Verification items for the finished model (mm, model axes). Face numbers are marked on the shaded views. A direction names the side the tool comes from. Round coordinates to 2 decimals unless told otherwise and drop trailing zeros. Order: outer loops, then holes, each group sorted by start corner. A loop starts at its lowest first (then second) coordinate and runs counter-clockwise, first axis right, second up. Notation, with made-up numbers: (64.5, -21.5) -> (119.5, -21.5) arc R24 ccw to (119.5, 13.5) -> close; hole circle Ø7 at (81.25, 66). An arc over 180 degrees is marked (long way). Put each result on its own line as item: value.
from build123d import *

# Parameters (mm, degrees)
CROQUIS1_W               = 22
CROQUIS1_H               = 55.2
SALIENTE_EXTRUIR1_DEPTH  = 4
CROQUIS2_W               = 12.1
CROQUIS2_H               = 4
CORTAR_EXTRUIR1_DEPTH    = 9.6
CROQUIS3_W               = 12.1
CROQUIS3_H               = 4
CORTAR_EXTRUIR2_DEPTH    = 9.6
CORTAR_EXTRUIR3_DEPTH    = 16
CORTAR_EXTRUIR4_START    = -16
CORTAR_EXTRUIR4_DEPTH    = 16
CROQUIS9_W               = 11.778481694
CROQUIS9_H               = 4
CORTAR_EXTRUIR5_DEPTH    = 2
CROQUIS11_W              = 4.95
CROQUIS11_H              = 4
SALIENTE_EXTRUIR3_DEPTH  = 2
CROQUIS12_W              = 4
CROQUIS12_H              = 1.8
SALIENTE_EXTRUIR4_DEPTH  = 12.1
CROQUIS13_W              = 4.95
CROQUIS13_H              = 4
SALIENTE_EXTRUIR5_DEPTH  = 2
CROQUIS14_W              = 4
CROQUIS14_H              = 1.8
SALIENTE_EXTRUIR6_DEPTH  = 12.1
CROQUIS17_W              = 4
CROQUIS17_H              = 59.2
SALIENTE_EXTRUIR8_DEPTH  = 15
CROQUIS18_W              = 4
CROQUIS18_H              = 59.2
SALIENTE_EXTRUIR9_DEPTH  = 15
CROQUIS19_R              = 1.75
CORTAR_EXTRUIR6_DEPTH    = 11.5
CROQUIS20_R              = 8.8
CROQUIS20_R_2            = 8.901027098
CORTAR_EXTRUIR7_DEPTH    = 4
CROQUIS22_R              = 10
SALIENTE_EXTRUIR10_DEPTH = 6
CORTAR_EXTRUIR8_DEPTH    = 10
CROQUIS26_R              = 8.901027098
CROQUIS26_R_2            = 8.8
CORTAR_EXTRUIR9_DEPTH    = 2


with BuildPart() as part:
    # Croquis1 → Saliente-Extruir1 (new body)
    with BuildSketch(Plane.XY):
        with Locations((11, 27.6)):
            Rectangle(CROQUIS1_W, CROQUIS1_H)
    extrude(amount=SALIENTE_EXTRUIR1_DEPTH)

    # Croquis2 → Cortar-Extruir1 (cut)
    with BuildSketch(Plane(origin=(0, 55.2, 0), x_dir=(1, 0, 0), z_dir=(0, 1, 0))):
        with Locations((11, -2)):
            Rectangle(CROQUIS2_W, CROQUIS2_H)
    extrude(amount=-CORTAR_EXTRUIR1_DEPTH, mode=Mode.SUBTRACT)

    # Croquis3 → Cortar-Extruir2 (cut)
    with BuildSketch(Plane.XZ):
        with Locations((11, 2)):
            Rectangle(CROQUIS3_W, CROQUIS3_H)
    extrude(amount=-CORTAR_EXTRUIR2_DEPTH, mode=Mode.SUBTRACT)

    # Croquis5 → Cortar-Extruir3 (cut)
    with BuildSketch(Plane.XZ.offset(-9.6)):
        with BuildLine():
            Line((7.4, 4), (14.6, 4))
            ThreePointArc((14.6, 4), (16.401151853, 1.506649462), (17.05, -1.5))
            Line((17.05, -1.5), (4.95, -1.5))
            ThreePointArc((4.95, -1.5), (5.598848147, 1.506649462), (7.4, 4))
        make_face()
    extrude(amount=-CORTAR_EXTRUIR3_DEPTH, mode=Mode.SUBTRACT)

    # Croquis7 → Cortar-Extruir4 (cut)
    with BuildSketch(Plane(origin=(0, 45.6, 0), x_dir=(1, 0, 0), z_dir=(0, 1, 0)).offset(CORTAR_EXTRUIR4_START)):
        with BuildLine():
            Line((4.95, 1.5), (17.05, 1.5))
            ThreePointArc((17.05, 1.5), (16.401151853, -1.506649462), (14.6, -4))
            Line((14.6, -4), (7.4, -4))
            ThreePointArc((7.4, -4), (5.598848147, -1.506649462), (4.95, 1.5))
        make_face()
    extrude(amount=CORTAR_EXTRUIR4_DEPTH, mode=Mode.SUBTRACT)

    # Croquis9 → Cortar-Extruir5 (cut)
    with BuildSketch(Plane(origin=(0, 0, 0), x_dir=(-1, 0, 0), z_dir=(0, 0, -1))):
        with Locations((-11, 27.6)):
            Rectangle(CROQUIS9_W, CROQUIS9_H)
    extrude(amount=-CORTAR_EXTRUIR5_DEPTH, mode=Mode.SUBTRACT)

    # Croquis11 → Saliente-Extruir3 (add)
    with BuildSketch(Plane(origin=(0, 55.2, 0), x_dir=(1, 0, 0), z_dir=(0, 1, 0))):
        with Locations((2.475, -2)):
            Rectangle(CROQUIS11_W, CROQUIS11_H)
        with Locations((19.525, -2)):
            Rectangle(CROQUIS11_W, CROQUIS11_H)
    extrude(amount=SALIENTE_EXTRUIR3_DEPTH)

    # Croquis12 → Saliente-Extruir4 (add)
    with BuildSketch(Plane(origin=(4.95, 0, 0), x_dir=(0, 0, -1), z_dir=(1, 0, 0))):
        with Locations((-2, 56.3)):
            Rectangle(CROQUIS12_W, CROQUIS12_H)
    extrude(amount=SALIENTE_EXTRUIR4_DEPTH)

    # Croquis13 → Saliente-Extruir5 (add)
    with BuildSketch(Plane.XZ):
        with Locations((19.525, 2)):
            Rectangle(CROQUIS13_W, CROQUIS13_H)
        with Locations((2.475, 2)):
            Rectangle(CROQUIS13_W, CROQUIS13_H)
    extrude(amount=SALIENTE_EXTRUIR5_DEPTH)

    # Croquis14 → Saliente-Extruir6 (add)
    with BuildSketch(Plane(origin=(4.95, 0, 0), x_dir=(0, 0, -1), z_dir=(1, 0, 0))):
        with Locations((-2, -1.1)):
            Rectangle(CROQUIS14_W, CROQUIS14_H)
    extrude(amount=SALIENTE_EXTRUIR6_DEPTH)

    # Croquis17 → Saliente-Extruir8 (add)
    with BuildSketch(Plane.ZY):
        with Locations((2, 27.6)):
            Rectangle(CROQUIS17_W, CROQUIS17_H)
    extrude(amount=SALIENTE_EXTRUIR8_DEPTH)

    # Croquis18 → Saliente-Extruir9 (add)
    with BuildSketch(Plane(origin=(22, 0, 0), x_dir=(0, 0, -1), z_dir=(1, 0, 0))):
        with Locations((-2, 27.6)):
            Rectangle(CROQUIS18_W, CROQUIS18_H)
    extrude(amount=SALIENTE_EXTRUIR9_DEPTH)

    # Croquis19 → Cortar-Extruir6 (cut)
    with BuildSketch(Plane(origin=(0, 0, 0), x_dir=(-1, 0, 0), z_dir=(0, 0, -1))):
        with Locations((-23.2, 54.9)):
            Circle(CROQUIS19_R)
        with Locations((1.2, 54)):
            Circle(CROQUIS19_R)
        with Locations((1.2, 0.5)):
            Circle(CROQUIS19_R)
        with Locations((-23.2, 0.5)):
            Circle(CROQUIS19_R)
    extrude(amount=-CORTAR_EXTRUIR6_DEPTH, mode=Mode.SUBTRACT)

    # Croquis20 → Cortar-Extruir7 (cut)
    with BuildSketch(Plane(origin=(0, 0, 0), x_dir=(-1, 0, 0), z_dir=(0, 0, -1))):
        with Locations((5, 27.6)):
            Circle(CROQUIS20_R)
        with Locations((-27, 27.6)):
            Circle(CROQUIS20_R_2)
    extrude(amount=-CORTAR_EXTRUIR7_DEPTH, mode=Mode.SUBTRACT)

    # Croquis22 → Saliente-Extruir10 (add)
    with BuildSketch(Plane.XY.offset(4)):
        with Locations(Location((-5, 27.6, 0), (0, 0, 180))):
            Circle(CROQUIS22_R)
        with Locations((27, 27.6)):
            Circle(CROQUIS22_R)
    extrude(amount=SALIENTE_EXTRUIR10_DEPTH)

    # Croquis25 → Cortar-Extruir8 (cut)
    with BuildSketch(Plane(origin=(0, 0, 0), x_dir=(-1, 0, 0), z_dir=(0, 0, -1))):
        Polygon((-27.444270401, 57.2), (-37, 34.275770323), (-37, 57.2), align=None)
        Polygon((5.217973102, 57.2), (15, 34.275770323), (15, 57.2), align=None)
        Polygon((-37, 20.547067511), (-27.444270401, -2), (-37, -2), align=None)
        Polygon((5.217973102, -2), (15, 22.810040502), (15, -2), align=None)
    extrude(amount=-CORTAR_EXTRUIR8_DEPTH, mode=Mode.SUBTRACT)

    # Croquis26 → Cortar-Extruir9 (cut)
    with BuildSketch(Plane(origin=(0, 0, 4), x_dir=(-1, 0, 0), z_dir=(0, 0, -1))):
        with Locations((-27, 27.6)):
            Circle(CROQUIS26_R)
        with Locations((5, 27.6)):
            Circle(CROQUIS26_R_2)
    extrude(amount=-CORTAR_EXTRUIR9_DEPTH, mode=Mode.SUBTRACT)

    # Croquis27 → Cortar-Revolución1 (revolve, cut)
    with BuildSketch(Plane(origin=(0, 0, 6), x_dir=(-1, 0, 0), z_dir=(0, 0, -1))):
        with BuildLine():
            Line((5, 36.4), (5, 18.8))
            ThreePointArc((5, 18.8), (13.8, 27.6), (5, 36.4))
        make_face()
    revolve(axis=Axis((-5, 36.4, 6), (0, -1, 0)), mode=Mode.SUBTRACT)

    # Croquis28 → Cortar-Revolución2 (revolve, cut)
    with BuildSketch(Plane(origin=(0, 0, 6), x_dir=(-1, 0, 0), z_dir=(0, 0, -1))):
        with BuildLine():
            Line((-27, 36.501027098), (-27, 18.698972902))
            ThreePointArc((-27, 18.698972902), (-35.901027098, 27.6), (-27, 36.501027098))
        make_face()
    revolve(axis=Axis((27, 36.501027098, 6), (0, -1, 0)), mode=Mode.SUBTRACT)


solid = part.part
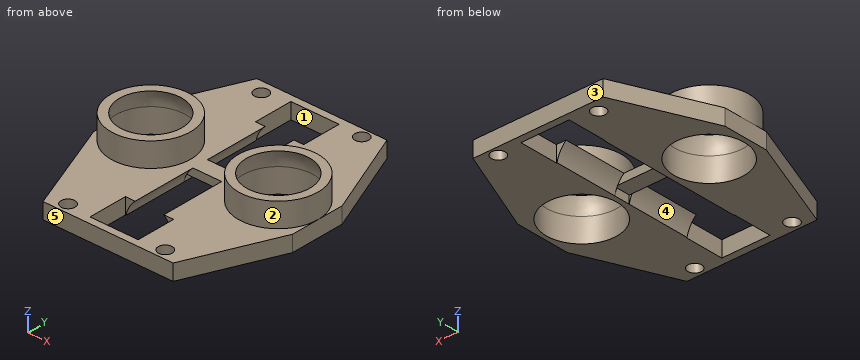
Item 1: Tool access check on the marked faces 1, 2, 3, 4 and 5. Record the directions out of +Z, -Z, +X, -X, +Y, -Y that give a thin tool (end or side, any length) a straight path to the whole face; none if there is none.
Check sheet entries:
face 1: +Z, -Z
face 2: +Z
face 3: +Z, -Z, +X, -X, +Y
face 4: -Z
face 5: +Z, -Z, +X, -X, -Y
Item 2: Section check B-B on y = 23.5. Record the boundary of the cut face in (x, z), then the cut area to 3 significant figures.
Check sheet entries:
outline: (-15, 0) -> (-12.79, 0) -> (-12.79, 6) arc R7.79 cw to (-11.68, 10) -> (-14.12, 10) -> (-14.12, 4) -> (-15, 4) -> close; (1.68, 10) arc R7.79 cw to (2.79, 6) -> (2.79, 0) -> (5.11, 0) arc R7.5 cw to (7.4, 4) -> (4.12, 4) -> (4.12, 10) -> close; (14.6, 4) arc R7.5 cw to (16.89, 0) -> (19.1, 0) -> (19.1, 6) arc R7.9 cw to (20.19, 10) -> (17.88, 10) -> (17.88, 4) -> close; (33.81, 10) arc R7.9 cw to (34.9, 6) -> (34.9, 0) -> (37, 0) -> (37, 4) -> (36.12, 4) -> (36.12, 10) -> close
area: 78.6 mm^2
Item 3: Section check C-C on z = 7.75. Record the boundary of the cut face in (x, y), then the cut area to 3 significant figures.
Check sheet entries:
outline: circle Ø20 at (-5, 27.6); circle Ø20 at (27, 27.6); hole circle Ø17.25 at (-5, 27.6); hole circle Ø17.45 at (27, 27.6)
area: 155 mm^2
Item 4: Material ranges on L1, parallel to X at y = 27.6, z = 3.35; L2, parallel to Y at x = 5.5, z = 3.25; L3, parallel to Y at x = 27, z = 4.6, recorded low to high. Write a range as [from, to].
Check sheet entries:
L1: x = [-15, -13.8], [3.8, 18.1], [35.9, 37]
L2: y = [-2, -0.2], [9.6, 45.6], [55.4, 57.2]
L3: y = [17.6, 18.7], [36.5, 37.6]
Item 5: Section check D-D on x = 23.2. Record the boundary of the cut face in (y, z), then the cut area to 3 significant figures.
Check sheet entries:
outline: (-2, 0) -> (-1.25, 0) -> (-1.25, 4) -> (-2, 4) -> close; (2.25, 0) -> (19.55, 0) -> (19.55, 6) arc R8.05 cw to (20.62, 10) -> (18.35, 10) -> (18.35, 4) -> (2.25, 4) -> close; (34.58, 10) arc R8.05 cw to (35.65, 6) -> (35.65, 0) -> (53.15, 0) -> (53.15, 4) -> (36.85, 4) -> (36.85, 10) -> close; (56.65, 0) -> (57.2, 0) -> (57.2, 4) -> (56.65, 4) -> close
area: 162 mm^2
Item 6: Section check A-A on x = -4. Record the boundary of the cut face in (y, z), then the cut area to 3 significant figures.
Check sheet entries:
outline: (-2, 0) -> (18.86, 0) -> (18.86, 6) arc R8.74 cw to (19.83, 10) -> (17.65, 10) -> (17.65, 4) -> (-2, 4) -> close; (35.37, 10) arc R8.74 cw to (36.34, 6) -> (36.34, 0) -> (57.2, 0) -> (57.2, 4) -> (37.55, 4) -> (37.55, 10) -> close
area: 184 mm^2
Item 7: Gauge pin test, flat ends, axial feed: pin 1 Ø23 at (x, y) = (27, 27.6) entering from +Z; pin 2 Ø1.5 at (x, y) = (16.5, 46.5) entering from +Z; pin 3 Ø4.5 at (x, y) = (9.5, 28.5) entering from -Z; pin 4 Ø3 at (y, z) = (50.5, 2) entering from +X. Record the tip position at first contact, or that the pin passes through.
Check sheet entries:
pin 1: stops at z = 10
pin 2: stops at z = 4
pin 3: stops at z = 2
pin 4: stops at x = 30.86
